For this review, use the dimensioned drawing (mm, ordinates from the lowest corner) and the shaded views. A direction names the side the tool comes from. Give positions to 0.01 mm unless a question says otherwise; leave off trailing zeros. Write each loop counter-clockwise with the first axis right and the second up, starting at its lowest first coordinate (ties: lowest second). Pieces come first, ordered by that corner, then holes. Notation, with made-up numbers: M 78,35 L 84,35 A6 cw 84,46 Z; hole C 57,12.25 d5. An arc over 180 degrees is marked long. Answer in a Markdown table with one row per item.
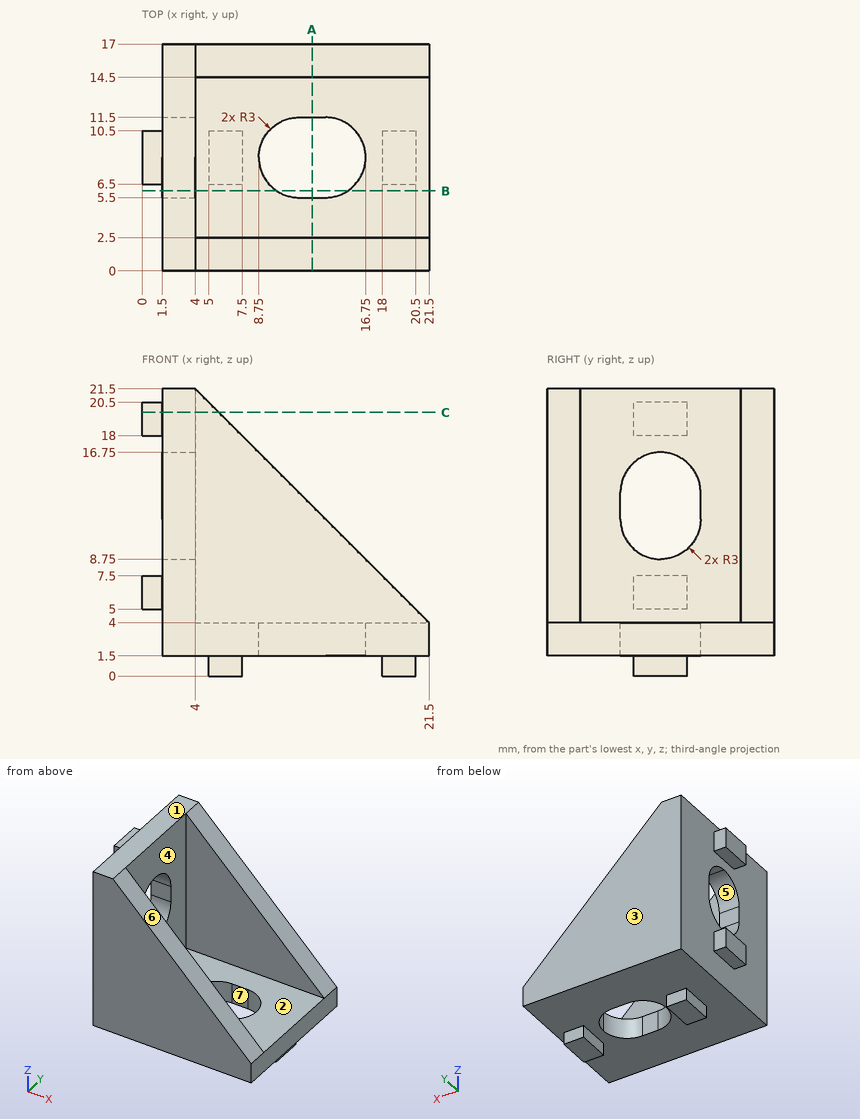
1) For the marked faces 4, 5, 6 and 7, list the 3-axis set-ups (+Z, -Z, +X, -X, +Y, -Y) from which the entire face can be reached by the end or side of a thin tool; tool diameter is ignored.
Geometry says:
| item | result |
|---|---|
| face 4 | +Z, +X |
| face 5 | +X, -X |
| face 6 | +Z, +X, +Y, -Y |
| face 7 | +Z, -Z |
2) Add section A-A (x = 12.75). Write out the cut boundary in (y, z), and give its area (4 significant figures).
Geometry says:
| item | result |
|---|---|
| outline | M 0,1.5 L 5.5,1.5 L 5.5,4 L 2.5,4 L 2.5,12.75 L 0,12.75 Z; M 11.5,1.5 L 17,1.5 L 17,12.75 L 14.5,12.75 L 14.5,4 L 11.5,4 Z |
| area | 71.25 mm^2 |
3) Insertion check: P1, Ø8, axis at y = 4, z = 14, coming from the -X side; P2, Ø1.6, axis at x = 0.5, z = 19.5, coming from the +Y side; P3, Ø2, axis at y = 4, z = 13, coming from the +X side. Each pin has a flat end and moves straight along its axis. Give the tip position at first contact, or say it passes through.
Geometry says:
| item | result |
|---|---|
| P1 | x = 1.5 |
| P2 | y = 10.5 |
| P3 | x = 4 |
4) Add section C-C (z = 19.75). Write out the cut boundary in (x, y), and give its area (4 significant figures).
Geometry says:
| item | result |
|---|---|
| outline | M 0,6.5 L 1.5,6.5 L 1.5,0 L 5.75,0 L 5.75,2.5 L 4,2.5 L 4,14.5 L 5.75,14.5 L 5.75,17 L 1.5,17 L 1.5,10.5 L 0,10.5 Z |
| area | 57.25 mm^2 |
5) Add section B-B (y = 6). Write out the cut boundary in (x, z), and give its area (3 significant figures).
Geometry says:
| item | result |
|---|---|
| outline | M 1.5,1.5 L 10.09,1.5 L 10.09,4 L 4,4 L 4,10.09 L 1.5,10.09 Z; M 1.5,15.41 L 4,15.41 L 4,21.5 L 1.5,21.5 Z; M 15.41,1.5 L 21.5,1.5 L 21.5,4 L 15.41,4 Z |
| area | 67.2 mm^2 |
6) To check wall thickness, follow probe 1 along Y at (x, z) = (14, 4.75); probe 2 along Z at (x, y) = (12.75, 4.25); probe 3 along X at (y, z) = (7, 1.25). State the ranges of each line that lie inside material, in increasing order. Write a range as [from, to].
Geometry says:
| item | result |
|---|---|
| probe 1 | [0, 2.5], [14.5, 17] |
| probe 2 | [1.5, 4] |
| probe 3 | [5, 7.5], [18, 20.5] |
7) The part is to be moulded in two halves that separate along Y. For the marked faces 1, 2 and 3, say which applies: released by +Y, released by -Y, zero draft, split by the parting line, or undercut.
Geometry says:
| item | result |
|---|---|
| face 1 | zero draft |
| face 2 | undercut |
| face 3 | released by +Y |
